The listing builds one solid part. Answer for the finished solid, in the listing's coordinates (mm). Face numbers are marked on the shaded views. Give positions to 0.01 mm unless a question says otherwise; leave off trailing zeros. Order: outer loops, then holes, each group sorted by start corner. A loop starts at its lowest first (then second) coordinate and runs counter-clockwise, first axis right, second up. Notation, with made-up numbers: (-34.75, 10) - (-15.75, 10) arc R20 cw to (-15.75, 28) - close; hole circle Ø9 at (34, 18). An arc over 180 degrees is marked (long way). Use a Markdown table: item, result. Add a question column.
1) Find section B-B, the plane z = 10.25. Determine the outline of the cut face in (x, y), plus the area to 3 significant figures.
2) Straight lines are drawn through the part: line 1 (Y direction, x = 0, z = 12.5); line 2 (Y direction, x = 16, z = 13.75); line 3 (X direction, y = -3.5, z = 15.75). For each, find the intervals that lie inside material, in ascending order.
3) Find section C-C, the plane x = 0. Determine the outline of the cut face in (y, z).
4) The mould has two halves that part along Y. Classify the marked faces 1, 2, 3 and 4: released by +Y, released by -Y, zero draft, split by the parting line, or undercut.
5) Find section A-A, the plane y = 0. Determine the outline of the cut face in (x, z), plus the area to 3 significant figures.
6) Flat-ended cylindrical pins translate along their axes: pin 1 (7 mm diameter, centred on x = 0, y = 0, fed in from -Z); pin 2 (5 mm diameter, centred on x = 15, y = 4, fed in from -Z). Find the tip coordinate at first contact, or state that the pin passes through.
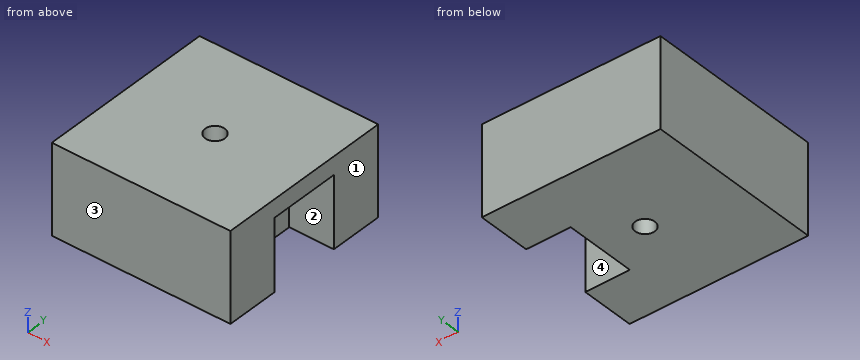
from build123d import *

# Parameters (mm, degrees)
F0_W     = 40
F0_H     = 40
F1_DEPTH = 20
F2_W     = 16
F2_H     = 16
F3_DEPTH = 10
F5_D     = 4.4


with BuildPart() as f1:
    # F0 (on Top) → F1 (new body)
    with BuildSketch(Plane.XY):
        Rectangle(F0_W, F0_H)
    extrude(amount=F1_DEPTH)

    # F2 (on face) → F3 (cut)
    with BuildSketch(Plane.YZ.offset(20)):
        with Locations((0, 8)):
            Rectangle(F2_W, F2_H)
    extrude(amount=-F3_DEPTH, mode=Mode.SUBTRACT)

    # F5 (through all)
    with Locations(Plane.XY.offset(20)):
        with Locations((0, 0)):
            Hole(F5_D / 2)


solid = f1.part
The answers:
| question | item | result |
|---|---|---|
| 1 | outline | (-20, -20) - (20, -20) - (20, -8) - (10, -8) - (10, 8) - (20, 8) - (20, 20) - (-20, 20) - close; hole circle Ø4.4 at (0, 0) |
| 1 | area | 1,420 mm2 |
| 2 | line 1 | -20 to -2.2, 2.2 to 20 |
| 2 | line 2 | -20 to -8, 8 to 20 |
| 2 | line 3 | -20 to 10 |
| 3 | outline | (-20, 0) - (-2.2, 0) - (-2.2, 20) - (-20, 20) - close; (2.2, 0) - (20, 0) - (20, 20) - (2.2, 20) - close |
| 4 | face 1 | zero draft |
| 4 | face 2 | undercut |
| 4 | face 3 | released by -Y |
| 4 | face 4 | undercut |
| 5 | outline | (-20, 0) - (-2.2, 0) - (-2.2, 20) - (-20, 20) - close; (2.2, 0) - (10, 0) - (10, 16) - (20, 16) - (20, 20) - (2.2, 20) - close |
| 5 | area | 552 mm2 |
| 6 | pin 1 | z = 0 |
| 6 | pin 2 | z = 16 |
